from build123d import *

# Parameters (mm, degrees)
SKETCH1_W              = 55
SKETCH1_H              = 40
BOSS_EXTRUDE1_DEPTH    = 5.6
M2_5_CLEARANCE_HOLE1_D = 2.9
SKETCH5_W              = 25
SKETCH5_H              = 7.4
BOSS_EXTRUDE2_DEPTH    = 14
SKETCH6_W              = 6
SKETCH6_H              = 20.5
BOSS_EXTRUDE3_DEPTH    = 8.5
CUT_EXTRUDE1_REACH     = 48.523
SKETCH8_W              = 35
SKETCH8_H              = 6
BOSS_EXTRUDE4_DEPTH    = 8.5
CUT_EXTRUDE2_REACH     = 61.501
SKETCH10_W             = 22
SKETCH10_H             = 9.5
BOSS_EXTRUDE5_DEPTH    = 12
BOSS_EXTRUDE6_DEPTH    = 4.5
LPATTERN1_COUNT        = 3
LPATTERN1_PITCH        = 12
SKETCH12_W             = 7.75
SKETCH12_H             = 9
BOSS_EXTRUDE7_DEPTH    = 3.9


with BuildPart() as part:
    # Sketch1 → Boss-Extrude1 (new body)
    with BuildSketch(Plane(origin=(0, 0, 0), x_dir=(1, 0, 0), z_dir=(0, 1, 0))):
        Rectangle(SKETCH1_W, SKETCH1_H)
    extrude(amount=BOSS_EXTRUDE1_DEPTH)

    # M2.5 Clearance Hole1 (through all)
    with Locations(Plane(origin=(0, 5.6, 0), x_dir=(-1, 0, 0), z_dir=(0, 1, 0))):
        with Locations((23.5, -16), (-23.5, 16)):
            Hole(M2_5_CLEARANCE_HOLE1_D / 2)

    # Sketch5 → Boss-Extrude2 (add)
    with BuildSketch(Plane(origin=(0, 5.6, 0), x_dir=(1, 0, 0), z_dir=(0, 1, 0))):
        with Locations((7.4, -15)):
            Rectangle(SKETCH5_W, SKETCH5_H)
    extrude(amount=BOSS_EXTRUDE2_DEPTH)

    # Sketch6 → Boss-Extrude3 (add)
    with BuildSketch(Plane(origin=(0, 5.6, 0), x_dir=(1, 0, 0), z_dir=(0, 1, 0))):
        with Locations((24.2, -1.75)):
            Rectangle(SKETCH6_W, SKETCH6_H)
    extrude(amount=BOSS_EXTRUDE3_DEPTH)

    # Sketch7 → Cut-Extrude1 (cut, up to next)
    with BuildSketch(Plane.XY.offset(12), mode=Mode.PRIVATE) as cut_extrude1_sk1:
        Polygon((25.7, 14.1), (27.2, 10), (27.2, 14.1), align=None)
    cut_extrude1_tool1 = extrude(cut_extrude1_sk1.sketch, amount=-CUT_EXTRUDE1_REACH, mode=Mode.PRIVATE) & part.part
    # Sketch7 → Cut-Extrude1 (cut, up to next)
    with BuildSketch(Plane.XY.offset(12), mode=Mode.PRIVATE) as cut_extrude1_sk2:
        Polygon((22.7, 14.1), (21.2, 10), (21.2, 14.1), align=None)
    cut_extrude1_tool2 = extrude(cut_extrude1_sk2.sketch, amount=-CUT_EXTRUDE1_REACH, mode=Mode.PRIVATE) & part.part
    add(cut_extrude1_tool1.solids().sort_by_distance((26.7, 12.733333, 12))[0], mode=Mode.SUBTRACT)
    add(cut_extrude1_tool2.solids().sort_by_distance((21.7, 12.733333, 12))[0], mode=Mode.SUBTRACT)

    # Sketch8 → Boss-Extrude4 (add)
    with BuildSketch(Plane(origin=(0, 5.6, 0), x_dir=(-1, 0, 0), z_dir=(0, 1, 0))):
        with Locations((-7.5, -16.7)):
            Rectangle(SKETCH8_W, SKETCH8_H)
    extrude(amount=BOSS_EXTRUDE4_DEPTH)

    # Sketch9 → Cut-Extrude2 (cut, up to next)
    with BuildSketch(Plane(origin=(25, 0, 0), x_dir=(0, 0, -1), z_dir=(1, 0, 0)), mode=Mode.PRIVATE) as cut_extrude2_sk1:
        Polygon((18.2, 14.1), (19.7, 10), (19.7, 14.1), align=None)
    cut_extrude2_tool1 = extrude(cut_extrude2_sk1.sketch, amount=-CUT_EXTRUDE2_REACH, mode=Mode.PRIVATE) & part.part
    # Sketch9 → Cut-Extrude2 (cut, up to next)
    with BuildSketch(Plane(origin=(25, 0, 0), x_dir=(0, 0, -1), z_dir=(1, 0, 0)), mode=Mode.PRIVATE) as cut_extrude2_sk2:
        Polygon((15.2, 14.1), (13.7, 10), (13.7, 14.1), align=None)
    cut_extrude2_tool2 = extrude(cut_extrude2_sk2.sketch, amount=-CUT_EXTRUDE2_REACH, mode=Mode.PRIVATE) & part.part
    add(cut_extrude2_tool1.solids().sort_by_distance((25, 12.733333, -19.2))[0], mode=Mode.SUBTRACT)
    add(cut_extrude2_tool2.solids().sort_by_distance((25, 12.733333, -14.2))[0], mode=Mode.SUBTRACT)

    # Sketch10 → Boss-Extrude5 (add)
    with BuildSketch(Plane(origin=(0, 5.6, 0), x_dir=(1, 0, 0), z_dir=(0, 1, 0))):
        with Locations((7.4, -5.05)):
            Rectangle(SKETCH10_W, SKETCH10_H)
    extrude(amount=BOSS_EXTRUDE5_DEPTH)

    # Sketch11 → Boss-Extrude6 (add)
    with BuildSketch(Plane(origin=(0, 5.6, 0), x_dir=(-1, 0, 0), z_dir=(0, 1, 0))):
        with BuildLine():
            Line((-19.2, -3.114213562), (-19.2, -8.871572875))
            Line((-19.2, -8.871572875), (-16.371572875, -11.7))
            Line((-16.371572875, -11.7), (-10.614213562, -11.7))
            Line((-10.614213562, -11.7), (-9.2, -10.285786438))
            Line((-9.2, -10.285786438), (-9.2, -4.528427125))
            Line((-9.2, -4.528427125), (-12.028427125, -1.7))
            Line((-12.028427125, -1.7), (-17.785786438, -1.7))
            ThreePointArc((-17.785786438, -1.7), (-18.785786438, -2.114213562), (-19.2, -3.114213562))
        make_face()
    boss_extrude6 = extrude(amount=BOSS_EXTRUDE6_DEPTH)

    # LPattern1: Boss-Extrude6 ×3
    with Locations(*[(-i * LPATTERN1_PITCH, 0, 0) for i in range(1, LPATTERN1_COUNT)]):
        add(boss_extrude6)

    # Sketch12 → Boss-Extrude7 (add)
    with BuildSketch(Plane(origin=(0, 5.6, 0), x_dir=(-1, 0, 0), z_dir=(0, 1, 0))):
        with Locations((20.325, 15.5)):
            Rectangle(SKETCH12_W, SKETCH12_H)
    extrude(amount=BOSS_EXTRUDE7_DEPTH)


solid = part.part
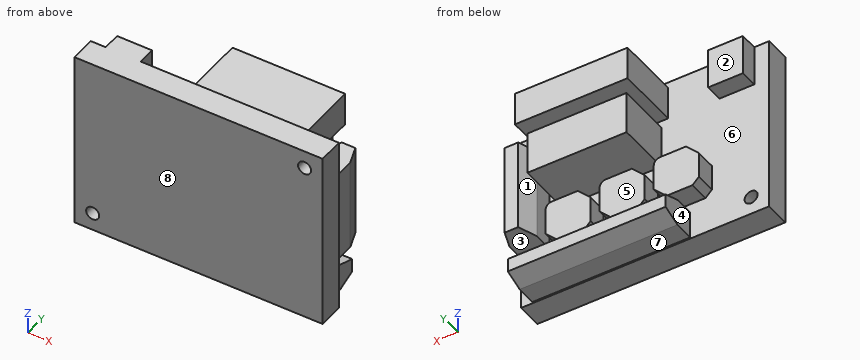
Read the model definition and answer for the solid it produces. Units are mm, in the model's axes. Face numbers are marked on the shaded views. A direction names the side the tool comes from. Round coordinates to 2 decimals unless told otherwise and drop trailing zeros. Order: outer loops, then holes, each group sorted by start corner. A loop starts at its lowest first (then second) coordinate and runs counter-clockwise, first axis right, second up. Notation, with made-up numbers: (-12, 21) - (30, 21) arc R16 ccw to (30, 49) - close; hole circle Ø3 at (54, 60.25). An arc over 180 degrees is marked (long way). Use one line per item in the form item = value. Start each with the question number.
(1) The part is cut by section D-D (y = 12). Give the vertices of the cut face in (x, z), then the cut area to 3 significant figures.
(2) Flat-ended cylindrical pins translate along their axes: pin 1 Ø8 at (x, z) = (4.5, -15) entering from +Y; pin 2 Ø2 at (y, z) = (8, -5) entering from +X; pin 3 Ø6 at (x, y) = (12, 10.5) entering from -Z. Find the tip coordinate at first contact, or state that the pin passes through.
(3) For the marked faces 1, 2, 3, 4 and 5, determine the directions among +Z, -Z, +X, -X, +Y, -Y from which every point of the face is accessible in a straight line to the end or side of a thin tool.
(4) Find the intervals of material crossed by line 1 along Z through (x, y) = (-23.5, 2.5); line 2 along Z through (x, y) = (23.5, 3.2); line 3 along Y through (x, z) = (-12, 9.5), in increasing order. Write a range as from..to.
(5) The part is cut by section B-B (x = 23.5). Give the vertices of the cut face in (y, z).
(6) The part is cut by section C-C (z = -16). Give the vertices of the cut face in (x, y).
(7) Determine the mould class of the marked faces 6, 7 and 8 for opening direction Z: +Z half, -Z half, draft (parallel to the pull), parting line (faces both ways), or undercut.
(8) The part is cut by section A-A (y = 14.75). Give the vertices of the cut face in (x, z), then the cut area to 3 significant figures.
Checked values:
q1.outline = (-10, -18.97) - (25, -18.97) - (25, -14.43) - (-10, -14.43) - close; (-5.1, 11.3) - (19.9, 11.3) - (19.9, 18.7) - (-5.1, 18.7) - close; (-3.6, 0.3) - (18.4, 0.3) - (18.4, 9.8) - (-3.6, 9.8) - close; (21.93, -8.5) - (26.47, -8.5) - (26.47, 12) - (21.93, 12) - close
q1.area = 646 mm^2
q2.pin_1 = 14.1
q2.pin_2 = 27.2
q2.pin_3 = -19.7
q3.face_1 = +Z, +Y
q3.face_2 = +Z, -Z, -X, +Y
q3.face_3 = +X, +Y
q3.face_4 = -Z, -X, +Y
q3.face_5 = -X, +Y
q4.line_1 = -20..-17.45, -14.55..20
q4.line_2 = -20..14.55, 17.45..20
q4.line_3 = 0..5.6
q5.outline = (0, -20) - (5.6, -20) - (5.6, -19.7) - (10, -19.7) - (14.1, -18.2) - (14.1, -15.2) - (10, -13.7) - (5.6, -13.7) - (5.6, -8.5) - (14.1, -8.5) - (14.1, 12) - (5.6, 12) - (5.6, 14.55) - (0, 14.55) - close; (0, 17.45) - (5.6, 17.45) - (5.6, 20) - (0, 20) - close
q6.outline = (-27.5, 0) - (-24.95, 0) - (-24.95, 5.6) - (-27.5, 5.6) - close; (-22.05, 0) - (27.5, 0) - (27.5, 5.6) - (25, 5.6) - (25, 14.1) - (-10, 14.1) - (-10, 5.6) - (-22.05, 5.6) - close
q7.face_6 = undercut
q7.face_7 = -Z half
q7.face_8 = draft
q8.outline = (-5.1, 11.3) - (19.9, 11.3) - (19.9, 18.7) - (-5.1, 18.7) - close; (-3.6, 0.3) - (18.4, 0.3) - (18.4, 9.8) - (-3.6, 9.8) - close
q8.area = 394 mm^2
